Geometry: see drawing. Coordinates: mm, zero at the bounding-box minimum. A direction names the side the tool comes from. Coordinates: 2 decimals unless noted, no trailing zeros. Order: outer loops, then holes, each group sorted by start corner. A loop starts at its lowest first (then second) coordinate and runs counter-clockwise, first axis right, second up.
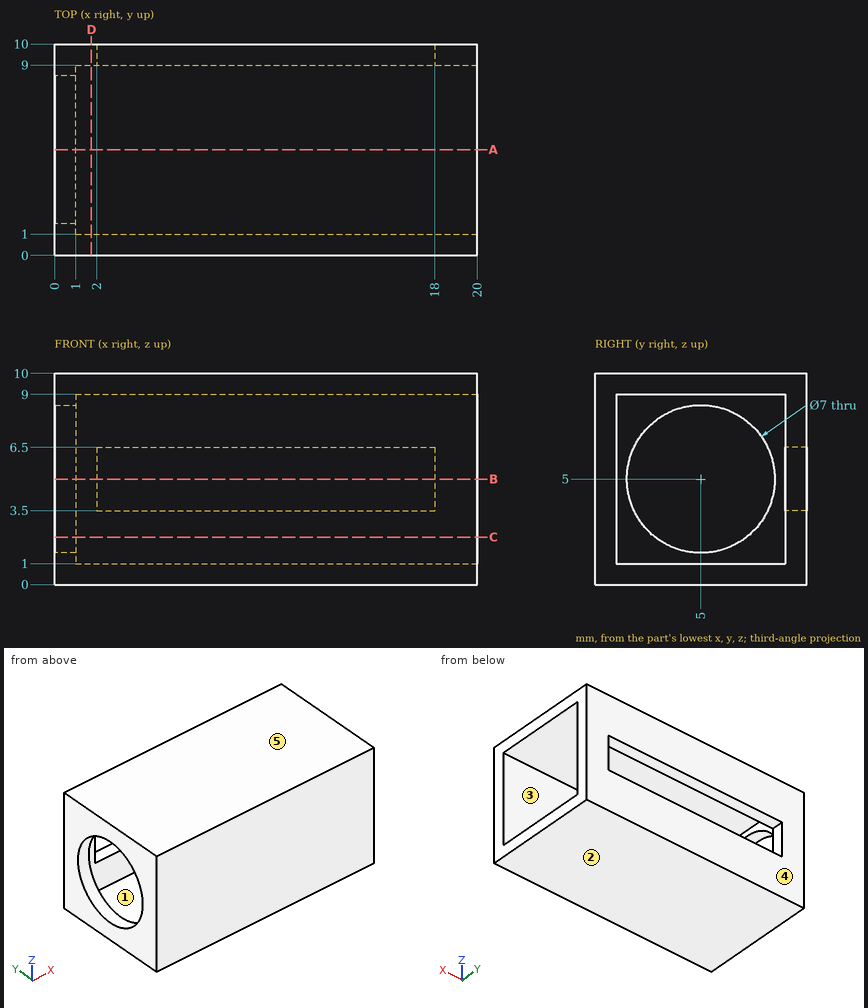
Q1. Material intervals for line 1 along Z through (x, y) = (13.5, 4); line 2 along Y through (x, z) = (0.65, 5), sorted ascending.
Solutions:
line 1: z = 0 to 1, 9 to 10
line 2: y = 0 to 1.5, 8.5 to 10
Q2. Section query B-B on z = 5. Output: boundary loops of the cut face in (x, y), plus the area to 3 significant figures.
Solutions:
outline: (0, 0) - (20, 0) - (20, 1) - (1, 1) - (1, 1.5) - (0, 1.5) - close; (0, 8.5) - (1, 8.5) - (1, 9) - (2, 9) - (2, 10) - (0, 10) - close; (18, 9) - (20, 9) - (20, 10) - (18, 10) - close
area: 25.0 mm2
Q3. Section query C-C on z = 2.25. Output: boundary loops of the cut face in (x, y), plus the area to 3 significant figures.
Solutions:
outline: (0, 0) - (20, 0) - (20, 1) - (1, 1) - (1, 2.83) - (0, 2.83) - close; (0, 7.17) - (1, 7.17) - (1, 9) - (20, 9) - (20, 10) - (0, 10) - close
area: 43.7 mm2
Q4. Section query D-D on x = 1.75. Output: boundary loops of the cut face in (y, z).
Solutions:
outline: (0, 0) - (10, 0) - (10, 10) - (0, 10) - close; hole (1, 1) - (9, 1) - (9, 9) - (1, 9) - close
Q5. Section query A-A on y = 5. Output: boundary loops of the cut face in (x, z).
Solutions:
outline: (0, 0) - (20, 0) - (20, 1) - (1, 1) - (1, 1.5) - (0, 1.5) - close; (0, 8.5) - (1, 8.5) - (1, 9) - (20, 9) - (20, 10) - (0, 10) - close
Q6. Pull-direction query (Y, two-part tool) for the marked faces 3, 4 and 5; classes: pulls with the +Y half, pulls with the -Y half, needs draft (parallel to the pull), parting line crosses it, or undercut.
Solutions:
face 3: undercut
face 4: pulls with the +Y half
face 5: needs draft
Q7. Pin query (flat end, axial travel): P1, Ø2.5, axis at y = 3.5, z = 6, coming from the +X side. Return the tip coordinate at first contact, or that it passes through.
Solutions:
P1: passes through
Q8. Set-up query: the marked faces 1 and 2. Return all of +Z, -Z, +X, -X, +Y, -Y with unobstructed straight access to the full face (end or side cutting, diameter ignored); none if empty.
Solutions:
face 1: +X
face 2: -Z, +X, -X, +Y, -Y
